Build history of the part. All positions in model axes, mm. Round coordinates to 2 decimals unless told otherwise and drop trailing zeros. Order: outer loops, then holes, each group sorted by start corner. A loop starts at its lowest first (then second) coordinate and runs counter-clockwise, first axis right, second up. Notation, with made-up numbers: (69, 16) -> (101, 16) arc R19 cw to (101, 47) -> close; hole circle Ø4 at (0.25, 73). An arc over 180 degrees is marked (long way). Use a Markdown table: item, result. Add a question column.
Item 1: Slice it at A-A, the plane x = -26.5. Give the cut face in (y, z), plus the area to 3 significant figures.
Item 2: Probe L1, parallel to Y at x = 26.5, z = 0.6; L2, parallel to Y at x = 51.5, z = 0.3; L3, parallel to Y at x = 73.5, z = 0.4. List the from-to ranges inside material, lowest first.
Item 3: Slice it at C-C, the plane y = 72.5. Give the cut face in (x, z).
Item 4: Slice it at B-B, the plane y = -64.5. Give the cut face in (x, z).
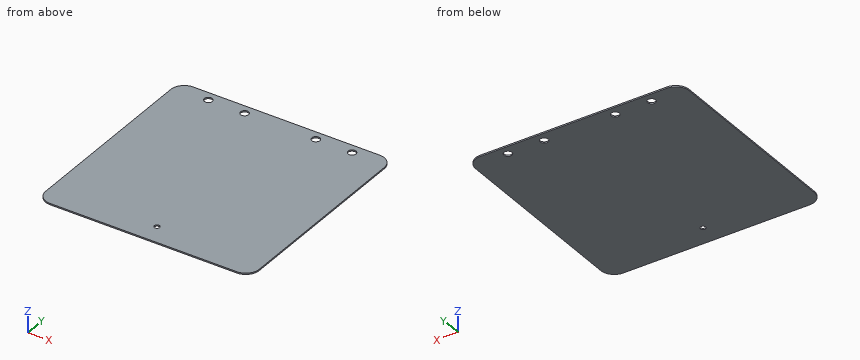
from build123d import *

# Parameters (mm, degrees)
EXTRUDE_1_DEPTH     = 1
SKETCH_2_R          = 3
CUT_EXTRUDE_1_DEPTH = 1
SKETCH_3_R          = 2
CUT_EXTRUDE_2_DEPTH = 1


with BuildPart() as part:
    # 스케치1 → 보스-돌출1 (new body)
    with BuildSketch(Plane.XY):
        with BuildLine():
            Line((-69.5, -79.5), (69.5, -79.5))
            ThreePointArc((69.5, -79.5), (76.571067812, -76.571067812), (79.5, -69.5))
            Line((79.5, -69.5), (79.5, 69.5))
            ThreePointArc((79.5, 69.5), (76.571067812, 76.571067812), (69.5, 79.5))
            Line((69.5, 79.5), (-69.5, 79.5))
            ThreePointArc((-69.5, 79.5), (-76.571067812, 76.571067812), (-79.5, 69.5))
            Line((-79.5, 69.5), (-79.5, -69.5))
            ThreePointArc((-79.5, -69.5), (-76.571067812, -76.571067812), (-69.5, -79.5))
        make_face()
    extrude(amount=EXTRUDE_1_DEPTH)

    # 스케치2 → 컷-돌출1 (cut)
    with BuildSketch(Plane.XY.offset(1)):
        with Locations((-53.5, 72.5)):
            Circle(SKETCH_2_R)
        with Locations((-26.5, 72.5)):
            Circle(SKETCH_2_R)
        with Locations((26.5, 72.5)):
            Circle(SKETCH_2_R)
        with Locations((53.5, 72.5)):
            Circle(SKETCH_2_R)
    extrude(amount=-CUT_EXTRUDE_1_DEPTH, mode=Mode.SUBTRACT)

    # 스케치3 → 컷-돌출2 (cut)
    with BuildSketch(Plane.XY.offset(1)):
        with Locations((0, -64.5)):
            Circle(SKETCH_3_R)
    extrude(amount=-CUT_EXTRUDE_2_DEPTH, mode=Mode.SUBTRACT)


solid = part.part
Check sheet entries:
| question | item | result |
|---|---|---|
| 1 | outline | (-79.5, 0) -> (69.5, 0) -> (69.5, 1) -> (-79.5, 1) -> close; (75.5, 0) -> (79.5, 0) -> (79.5, 1) -> (75.5, 1) -> close |
| 1 | area | 153 mm2 |
| 2 | L1 | -79.5 to 69.5, 75.5 to 79.5 |
| 2 | L2 | -79.5 to 70.26, 74.74 to 79.5 |
| 2 | L3 | -78.67 to 78.67 |
| 3 | outline | (-79.04, 0) -> (-56.5, 0) -> (-56.5, 1) -> (-79.04, 1) -> close; (-50.5, 0) -> (-29.5, 0) -> (-29.5, 1) -> (-50.5, 1) -> close; (-23.5, 0) -> (23.5, 0) -> (23.5, 1) -> (-23.5, 1) -> close; (29.5, 0) -> (50.5, 0) -> (50.5, 1) -> (29.5, 1) -> close; (56.5, 0) -> (79.04, 0) -> (79.04, 1) -> (56.5, 1) -> close |
| 4 | outline | (-79.5, 0) -> (-2, 0) -> (-2, 1) -> (-79.5, 1) -> close; (2, 0) -> (79.5, 0) -> (79.5, 1) -> (2, 1) -> close |
